Verification items for the finished model (mm, model axes). A direction names the side the tool comes from. Round coordinates to 2 decimals unless told otherwise and drop trailing zeros. Loops run counter-clockwise (first coordinate to the right, second up) from the corner with the lowest first, then second, coordinate; pieces in that order, holes last. Notation, with made-up numbers: (-28.5, -11) -> (10.5, -11) arc R9 ccw to (10.5, -6) -> close; hole circle Ø10 at (87, 71.5). An arc over 180 degrees is marked (long way). Use a Markdown table: item, result. Add a question column.
```python
from build123d import *

# Parameters (mm, degrees)
F1_DEPTH = 5.08
F2_DEPTH = 13.97
F3_START = 3.81
F3_DEPTH = 5.08
F4_R     = 3.048
F4_W     = 12.7
F4_H     = 6.985
F5_DEPTH = 5.08
F6_SIZE  = 1.524


with BuildPart() as f1:
    # F0 (on Top) → F1 (new body)
    with BuildSketch(Plane.XY):
        with BuildLine():
            ThreePointArc((-10.16, -0.9357894737), (-9.2602083301, 3.2444188564), (-6.7202083301, 6.6842105263))
            Line((-6.7202083301, 6.6842105263), (-17.78, 6.6842105263))
            Line((-17.78, 6.6842105263), (-17.78, -3.4757894737))
            Line((-17.78, -3.4757894737), (-10.16, -3.4757894737))
            Line((-10.16, -3.4757894737), (-10.16, -0.9357894737))
        make_face()
        with BuildLine():
            Line((17.78, 6.6842105263), (6.7202083301, 6.6842105263))
            ThreePointArc((6.7202083301, 6.6842105263), (9.2602083301, 3.2444188564), (10.16, -0.9357894737))
            Line((10.16, -0.9357894737), (10.16, -3.4757894737))
            Line((10.16, -3.4757894737), (17.78, -3.4757894737))
            Line((17.78, -3.4757894737), (17.78, 6.6842105263))
        make_face()
        with BuildLine():
            Line((-9.017, -3.4757894737), (-9.017, -0.9357894737))
            ThreePointArc((-9.017, -0.9357894737), (-7.8986424103, 3.4136630291), (-4.8209842356, 6.6842105263))
            Line((-4.8209842356, 6.6842105263), (-6.7202083301, 6.6842105263))
            ThreePointArc((-6.7202083301, 6.6842105263), (-9.2602083301, 3.2444188564), (-10.16, -0.9357894737))
            ThreePointArc((-10.16, -0.9357894737), (-10.0790217141, -2.2159930853), (-9.8373776994, -3.4757894737))
            Line((-9.8373776994, -3.4757894737), (-9.017, -3.4757894737))
        make_face()
        with BuildLine():
            ThreePointArc((4.8209842356, 6.6842105263), (7.8986424103, 3.4136630291), (9.017, -0.9357894737))
            Line((9.017, -0.9357894737), (9.017, -3.4757894737))
            Line((9.017, -3.4757894737), (9.8373776994, -3.4757894737))
            ThreePointArc((9.8373776994, -3.4757894737), (10.0790217141, -2.2159930853), (10.16, -0.9357894737))
            ThreePointArc((10.16, -0.9357894737), (9.2602083301, 3.2444188564), (6.7202083301, 6.6842105263))
            Line((6.7202083301, 6.6842105263), (4.8209842356, 6.6842105263))
        make_face()
        with BuildLine():
            ThreePointArc((-4.8209842356, 6.6842105263), (0, 8.0812105263), (4.8209842356, 6.6842105263))
            Line((4.8209842356, 6.6842105263), (6.7202083301, 6.6842105263))
            ThreePointArc((6.7202083301, 6.6842105263), (0, 9.2242105263), (-6.7202083301, 6.6842105263))
            Line((-6.7202083301, 6.6842105263), (-4.8209842356, 6.6842105263))
        make_face()
        with BuildLine():
            Line((-10.16, -3.4757894737), (-9.8373776994, -3.4757894737))
            ThreePointArc((-9.8373776994, -3.4757894737), (-10.0790217141, -2.2159930853), (-10.16, -0.9357894737))
            Line((-10.16, -0.9357894737), (-10.16, -3.4757894737))
        make_face()
        with BuildLine():
            ThreePointArc((10.16, -0.9357894737), (10.0790217141, -2.2159930853), (9.8373776994, -3.4757894737))
            Line((9.8373776994, -3.4757894737), (10.16, -3.4757894737))
            Line((10.16, -3.4757894737), (10.16, -0.9357894737))
        make_face()
    extrude(amount=-F1_DEPTH)

    # F0 (on Top) → F2 (join)
    with BuildSketch(Plane.XY):
        with BuildLine():
            ThreePointArc((-6.7202083301, 6.6842105263), (0, 9.2242105263), (6.7202083301, 6.6842105263))
            Line((6.7202083301, 6.6842105263), (17.78, 6.6842105263))
            Line((17.78, 6.6842105263), (17.78, -3.4757894737))
            Line((17.78, -3.4757894737), (22.86, -3.4757894737))
            Line((22.86, -3.4757894737), (22.86, 11.7642105263))
            Line((22.86, 11.7642105263), (-22.86, 11.7642105263))
            Line((-22.86, 11.7642105263), (-22.86, -3.4757894737))
            Line((-22.86, -3.4757894737), (-17.78, -3.4757894737))
            Line((-17.78, -3.4757894737), (-17.78, 6.6842105263))
            Line((-17.78, 6.6842105263), (-6.7202083301, 6.6842105263))
        make_face()
    extrude(amount=-F2_DEPTH)

    # F1_face (on face) → F3 (join)
    with BuildSketch(Plane(origin=(0, 2.3290563147, -5.08), x_dir=(1, 0, 0), z_dir=(0, 0, -1)).offset(F3_START)):
        with BuildLine():
            Line((-17.78, 5.8048457884), (-17.78, -4.3551542116))
            Line((-17.78, -4.3551542116), (-6.7202083301, -4.3551542116))
            ThreePointArc((-6.7202083301, -4.3551542116), (0, -6.8951542116), (6.7202083301, -4.3551542116))
            Line((6.7202083301, -4.3551542116), (17.78, -4.3551542116))
            Line((17.78, -4.3551542116), (17.78, 5.8048457884))
            Line((17.78, 5.8048457884), (9.017, 5.8048457884))
            Line((9.017, 5.8048457884), (9.017, 3.2648457884))
            ThreePointArc((9.017, 3.2648457884), (0, -5.7521542116), (-9.017, 3.2648457884))
            Line((-9.017, 3.2648457884), (-9.017, 5.8048457884))
            Line((-9.017, 5.8048457884), (-17.78, 5.8048457884))
        make_face()
    extrude(amount=F3_DEPTH)

    # F4 (on face) → F5 (join)
    with BuildSketch(Plane(origin=(0, 11.7642105263, 0), x_dir=(-1, 0, 0), z_dir=(0, 1, 0))):
        Polygon((12.7, 0), (12.7, 31.115), (-12.7, 31.115), (-12.7, 0), (0, 0), align=None)
        with Locations((0, 23.1394)):
            Circle(F4_R, mode=Mode.SUBTRACT)
        Polygon((12.7, -45.085), (12.7, -13.97), (0, -13.97), (-12.7, -13.97), (-12.7, -45.085), align=None)
        with Locations((0, -37.1094)):
            Circle(F4_R, mode=Mode.SUBTRACT)
        with Locations((6.35, -10.4775)):
            Rectangle(F4_W, F4_H)
        Polygon((0, -6.985), (0, 0), (-12.7, 0), (-12.7, -13.97), (0, -13.97), align=None)
        with Locations((6.35, -3.4925)):
            Rectangle(F4_W, F4_H)
    extrude(amount=F5_DEPTH)

    # F6
    f6_edges = [f1.edges().sort_by_distance(p)[0] for p in [
        (3.048, 11.764211, 23.1394),
        (3.048, 11.764211, -37.1094),
    ]]
    chamfer(f6_edges, length=F6_SIZE)


solid = f1.part
```
1) Sectioned sample at C-C on z = -6. Enter the section's corners in (x, y).
2) Sectioned sample at D-D on x = 19.5. Enter the section's corners in (y, z).
3) Thickness scan on line 1 (Z direction, x = 0, y = 14.5) (3 decimals); line 2 (X direction, y = -2.5, z = -0.5); line 3 (Z direction, x = -15.5, y = 1.75). Record the ranges inside material, lowest first.
4) Access from +Z, -Z, +X, -X, +Y, -Y to the whole of each face (thin tool, end or side, straight path). Record for faces 1 (the face through (0, 11.764, -29)), 2 (the face through (0, 9, -5.08)), 3 (the face through (0, 11.764, 16)).
5) Go/stop test with flat-tipped pins: pin 1 (4.5 mm diameter, centred on x = -6.5, y = 1.5, fed in from +Z); pin 2 (2.5 mm diameter, centred on y = 14, z = -7, fed in from +X); pin 3 (1.9 mm diameter, centred on x = 12, z = -7, fed in from -Y); pin 4 (5 mm diameter, centred on x = 0, z = -37.11, fed in from -Y). Record where each tip stops, or that it passes through.
6) Release check for a two-part mould opening along X. For faces 4 (the face through (12, 6.684, -7)), 5 (the face through (-12.7, 14, -8)), 6 (the face through (-19, -3.476, -7)) record: released by +X, released by -X, zero draft, split by the parting line, or undercut.
7) Sectioned sample at A-A on x = 0. Enter the section's corners in (y, z) (3 decimals), then the cut area to 3 significant figures.
8) Sectioned sample at B-B on y = 5.25. Enter the section's corners in (x, z).
Geometry results:
| question | item | result |
|---|---|---|
| 1 | outline | (-22.86, -3.48) -> (-17.78, -3.48) -> (-17.78, 6.68) -> (-6.72, 6.68) arc R10.16 cw to (6.72, 6.68) -> (17.78, 6.68) -> (17.78, -3.48) -> (22.86, -3.48) -> (22.86, 11.76) -> (12.7, 11.76) -> (12.7, 16.84) -> (-12.7, 16.84) -> (-12.7, 11.76) -> (-22.86, 11.76) -> close |
| 2 | outline | (-3.48, -13.97) -> (11.76, -13.97) -> (11.76, 0) -> (-3.48, 0) -> close |
| 3 | line 1 | -45.085 to -40.157, -34.061 to 20.091, 26.187 to 31.115 |
| 3 | line 2 | -22.86 to -9.02, 9.02 to 22.86 |
| 3 | line 3 | -13.97 to -8.89, -5.08 to 0 |
| 4 | face 1 | -Z, +X, -X, -Y |
| 4 | face 2 | -Y |
| 4 | face 3 | +Z, +X, -X, -Y |
| 5 | pin 1 | z = 0 |
| 5 | pin 2 | x = 12.7 |
| 5 | pin 3 | y = 6.68 |
| 5 | pin 4 | through |
| 6 | face 4 | undercut |
| 6 | face 5 | released by -X |
| 6 | face 6 | zero draft |
| 7 | outline | (8.081, -13.97) -> (11.764, -13.97) -> (11.764, -32.537) -> (13.288, -34.061) -> (16.844, -34.061) -> (16.844, 20.091) -> (13.288, 20.091) -> (11.764, 18.567) -> (11.764, 0) -> (8.081, 0) -> (8.081, -5.08) -> (9.224, -5.08) -> (9.224, -8.89) -> (8.081, -8.89) -> close; (11.764, -45.085) -> (16.844, -45.085) -> (16.844, -40.157) -> (13.288, -40.157) -> (11.764, -41.681) -> close; (11.764, 27.711) -> (13.288, 26.187) -> (16.844, 26.187) -> (16.844, 31.115) -> (11.764, 31.115) -> close |
| 7 | area | 368 mm^2 |
| 8 | outline | (-22.86, -13.97) -> (-6.56, -13.97) -> (-6.56, -8.89) -> (-17.78, -8.89) -> (-17.78, -5.08) -> (-6.56, -5.08) -> (-6.56, 0) -> (-22.86, 0) -> close; (6.56, -13.97) -> (22.86, -13.97) -> (22.86, 0) -> (6.56, 0) -> (6.56, -5.08) -> (17.78, -5.08) -> (17.78, -8.89) -> (6.56, -8.89) -> close |
